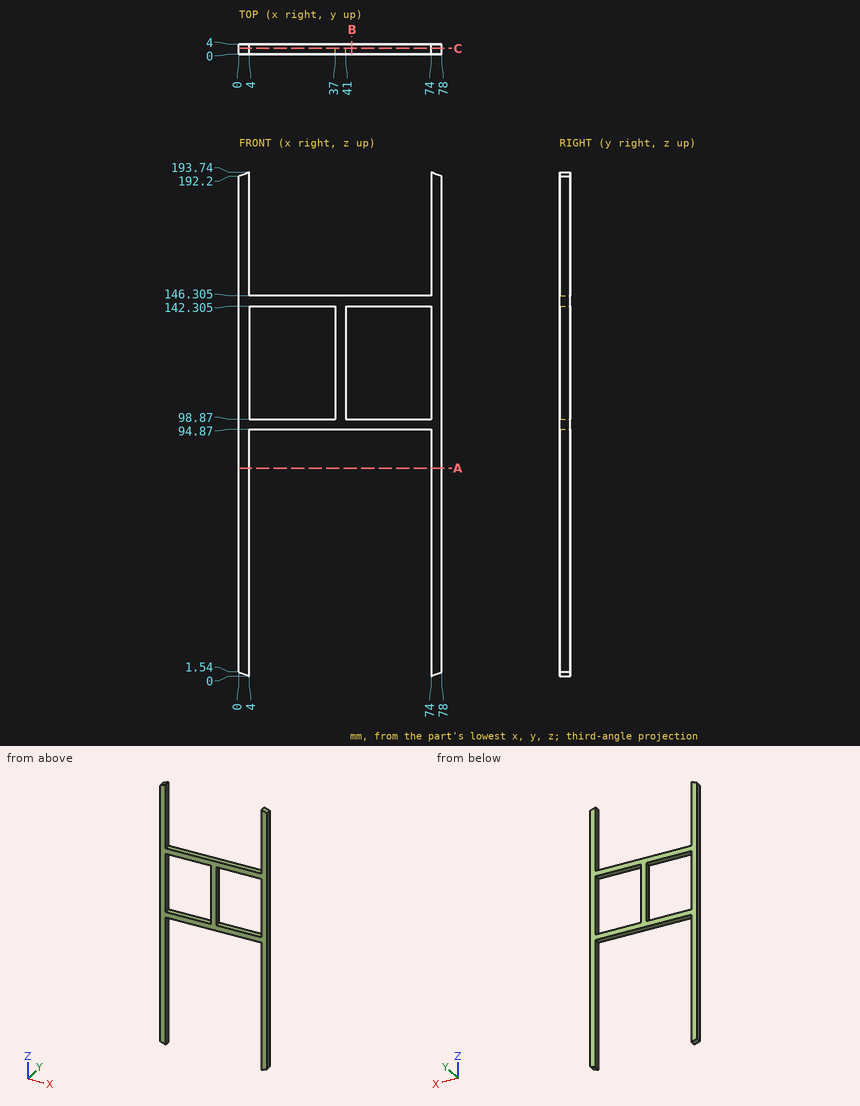
Study the drawing (mm; zero at the part's minimum x, y, z) and answer. Give positions to 0.01 mm unless a question says otherwise; leave off trailing zeros. Write each loop counter-clockwise with the first axis right and the second up, starting at its lowest first coordinate (ties: lowest second). Pieces come first, ordered by that corner, then holes. Notation, with made-up numbers: (5.25, -4) -> (60.25, -4) arc R10 ccw to (60.25, 5) -> close; hole circle Ø4 at (14.25, 36.5). An arc over 180 degrees is marked (long way). Answer as a JSON object with one key per item and string values. Group by question number.
1) Find section B-B (x = 43.5). Write down the section's boundary in (y, z) (3 decimals).
2) Find section A-A (z = 80). Write down the section's boundary in (x, y).
3) Consider L1, parallel to Z at x = 28, y = 1.6 (3 decimals); L2, parallel to X at y = 1.9, z = 20. Determine where each line is inside the solid, lowest interval first. Write a range as from..to.
4) Find section C-C (y = 2.3). Write down the section's boundary in (x, z) (3 decimals), and give its area (3 significant figures).
5) Each of these flat-tipped pins is pushed along its axis until it touches: P1, Ø2, axis at x = 44, y = 2.5, coming from the -Z side; P2, Ø1.5, axis at x = 31.5, y = 1.5, coming from the +Z side (3 decimals). Where does it stop, or does it pass through?
Values follow:
{
 "1": {"outline": "(0, 94.87) -> (4, 94.87) -> (4, 98.87) -> (0, 98.87) -> close; (0, 142.305) -> (4, 142.305) -> (4, 146.305) -> (0, 146.305) -> close"},
 "2": {"outline": "(0, 0) -> (4, 0) -> (4, 4) -> (0, 4) -> close; (74, 0) -> (78, 0) -> (78, 4) -> (74, 4) -> close"},
 "3": {"L1": "z = 94.87..98.87, 142.305..146.305", "L2": "x = 0..4, 74..78"},
 "4": {"outline": "(0, 1.54) -> (4, 0) -> (4, 94.87) -> (74, 94.87) -> (74, 0) -> (78, 1.54) -> (78, 192.2) -> (74, 193.74) -> (74, 146.305) -> (4, 146.305) -> (4, 193.74) -> (0, 192.2) -> close; hole (4, 98.87) -> (37, 98.87) -> (37, 142.305) -> (4, 142.305) -> close; hole (41, 98.87) -> (74, 98.87) -> (74, 142.305) -> (41, 142.305) -> close", "area": "2,270 mm2"},
 "5": {"P1": "stops at z = 94.87", "P2": "stops at z = 146.305"}
}
